The drawing under review shows one solid part. Ordinate dimensions are in mm from its lowest x, y, z. A direction names the side the tool comes from. Round coordinates to 2 decimals unless told otherwise and drop trailing zeros. Loops run counter-clockwise (first coordinate to the right, second up) from the corner with the lowest first, then second, coordinate; pieces in that order, holes last. Notation, with made-up numbers: (-39.5, 23.25) - (-16.5, 23.25) arc R19 ccw to (-16.5, 43.25) - close; hole circle Ø10 at (43.5, -22.5). An arc over 180 degrees is marked (long way). Answer as CSV lines item,"result".
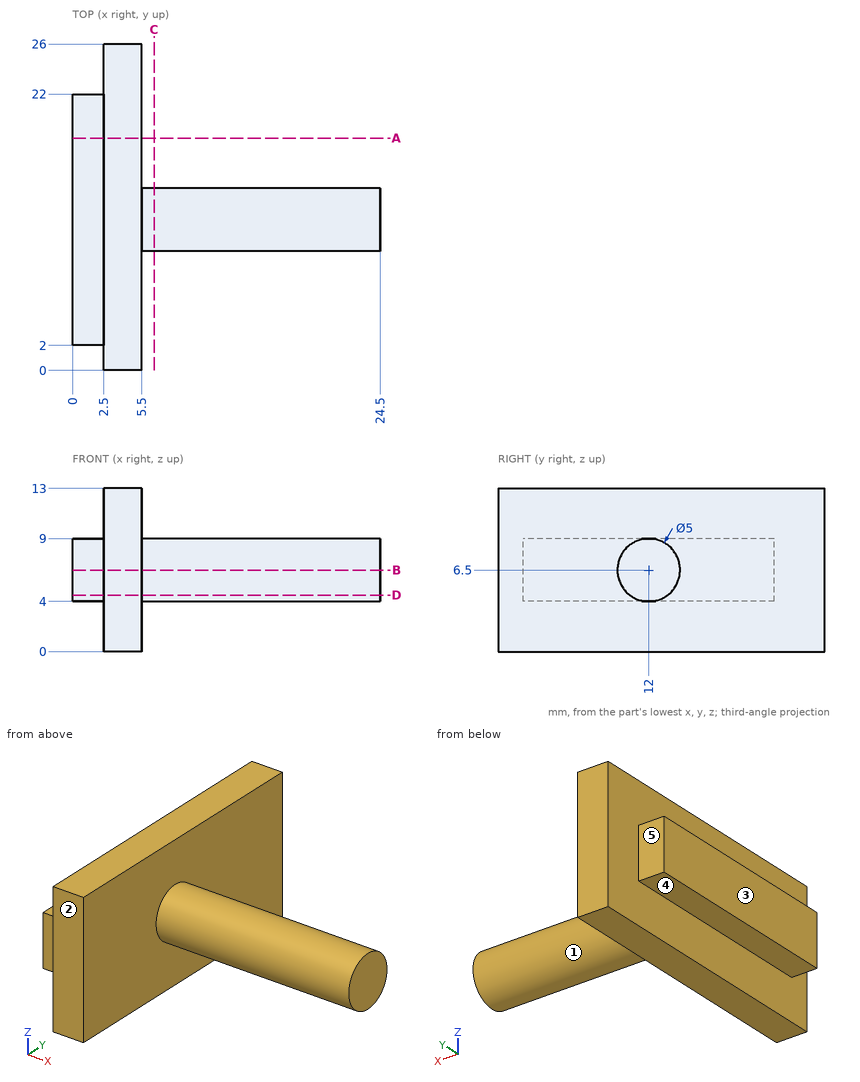
1. Take a section at B-B (z = 6.5). State the section outline as (x, y) points.
Numbers:
outline,"(0, 2) - (2.5, 2) - (2.5, 0) - (5.5, 0) - (5.5, 9.5) - (24.5, 9.5) - (24.5, 14.5) - (5.5, 14.5) - (5.5, 26) - (2.5, 26) - (2.5, 22) - (0, 22) - close"
2. Tool access review of the marked faces 1, 2, 3, 4 and 5: name each direction out of +Z, -Z, +X, -X, +Y, -Y from which nothing blocks a thin tool from reaching the whole face with its end or side.
Numbers:
face 1,"+X"
face 2,"+Z, -Z, +X, -X, -Y"
face 3,"+Z, -Z, -X, +Y, -Y"
face 4,"-Z, -X, +Y, -Y"
face 5,"+Z, -Z, -X, +Y"
3. Clearance check with flat-ended pins moving along their axes: pin 1 (1.2 mm diameter, centred on x = 1.5, y = 7.5, fed in from -Z); pin 2 (8 mm diameter, centred on x = 10.5, y = 12.5, fed in from +Z). State where each tip first meets the part, or that it passes through.
Numbers:
pin 1,"stops at z = 4"
pin 2,"stops at z = 9"
4. Take a section at C-C (x = 6.5). State the section outline as (y, z) points, plus the area to 3 significant figures.
Numbers:
outline,"circle Ø5 at (12, 6.5)"
area,"19.6 mm²"
5. Take a section at A-A (y = 18.5). State the section outline as (x, z) points.
Numbers:
outline,"(0, 4) - (2.5, 4) - (2.5, 0) - (5.5, 0) - (5.5, 13) - (2.5, 13) - (2.5, 9) - (0, 9) - close"
6. Take a section at D-D (z = 4.5). State the section outline as (x, y) points.
Numbers:
outline,"(0, 2) - (2.5, 2) - (2.5, 0) - (5.5, 0) - (5.5, 10.5) - (24.5, 10.5) - (24.5, 13.5) - (5.5, 13.5) - (5.5, 26) - (2.5, 26) - (2.5, 22) - (0, 22) - close"
7. Wall thickness on probe 1 along X at (y, z) = (7.25, 5.5); probe 2 along X at (y, z) = (1, 9.5); probe 3 along Z at (x, y) = (16.75, 9.75): over which ranges is each line inside the solid? List them lowest first.
Numbers:
probe 1,"x = 0 to 5.5"
probe 2,"x = 2.5 to 5.5"
probe 3,"z = 5.41 to 7.59"
